```python
from build123d import *

# Parameters (mm, degrees)
SKETCH1_W           = 18
SKETCH1_H           = 28
SKETCH1_W_2         = 13
SKETCH1_H_2         = 16.2
BOSS_EXTRUDE1_DEPTH = 3
SKETCH1_3_W         = 13
SKETCH1_3_H         = 16.2
CUT_EXTRUDE1_DEPTH  = 17.911534525
SKETCH2_W           = 16.25
SKETCH2_H           = 19.6
CUT_EXTRUDE2_DEPTH  = 2
SKETCH4_W           = 10
SKETCH4_H           = 9
CUT_EXTRUDE3_DEPTH  = 17.911534525


with BuildPart() as part:
    # Sketch1 → Boss-Extrude1 (new body)
    # profile 1 of 2: a face of its own
    with BuildSketch(Plane(origin=(0, 0, 0), x_dir=(1, 0, 0), z_dir=(0, 1, 0))):
        Rectangle(SKETCH1_W, SKETCH1_H)
        Rectangle(SKETCH1_W_2, SKETCH1_H_2, mode=Mode.SUBTRACT)
    # profile 2 of 2: a face of its own
    with BuildSketch(Plane(origin=(0, 0, 0), x_dir=(1, 0, 0), z_dir=(0, 1, 0))):
        Rectangle(SKETCH1_W_2, SKETCH1_H_2)
    extrude(amount=BOSS_EXTRUDE1_DEPTH)

    # Sketch1<3> → Cut-Extrude1 (cut, through all)
    with BuildSketch(Plane(origin=(0, 0, 0), x_dir=(1, 0, 0), z_dir=(0, 1, 0))):
        Rectangle(SKETCH1_3_W, SKETCH1_3_H)
    extrude(amount=CUT_EXTRUDE1_DEPTH, mode=Mode.SUBTRACT)

    # Sketch2 → Cut-Extrude2 (cut)
    with BuildSketch(Plane(origin=(0, 3, 0), x_dir=(1, 0, 0), z_dir=(0, 1, 0))):
        Rectangle(SKETCH2_W, SKETCH2_H)
    extrude(amount=-CUT_EXTRUDE2_DEPTH, mode=Mode.SUBTRACT)

    # Sketch4 → Cut-Extrude3 (cut, through all)
    with BuildSketch(Plane(origin=(0, 3, 0), x_dir=(1, 0, 0), z_dir=(0, 1, 0))):
        with Locations((0, 9.8)):
            Rectangle(SKETCH4_W, SKETCH4_H)
    extrude(amount=-CUT_EXTRUDE3_DEPTH, mode=Mode.SUBTRACT)


solid = part.part
```
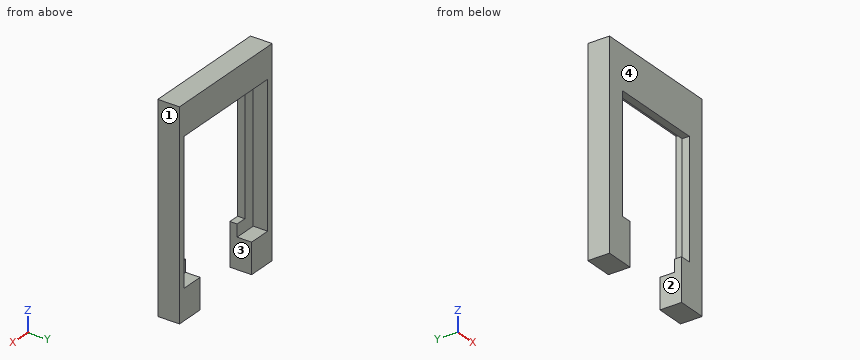
Verification items for the finished model (mm, model axes). Face numbers are marked on the shaded views. Give positions to 0.01 mm unless a question says otherwise; leave off trailing zeros. Order: outer loops, then holes, each group sorted by start corner. A loop starts at its lowest first (then second) coordinate and runs counter-clockwise, first axis right, second up. Notation, with made-up numbers: (81, 31) -> (122, 31) arc R22 cw to (122, 44) -> close; hole circle Ø10 at (-20, 79.5). An arc over 180 degrees is marked (long way). Use a Markdown table: item, result.
1) Section check C-C, the plane y = 2.2. Record the boundary of the cut face in (x, z) (3 decimals).
Results:
| item | result |
|---|---|
| outline | (-9, -14) -> (-5, -14) -> (-5, -9.8) -> (-8.125, -9.8) -> (-8.125, 9.8) -> (8.125, 9.8) -> (8.125, -9.8) -> (5, -9.8) -> (5, -14) -> (9, -14) -> (9, 14) -> (-9, 14) -> close |
2) Depth check by flat-ended pin: pin 1 Ø1.1 at (x, y) = (0, 0.5) entering from -Z; pin 2 Ø1.5 at (x, z) = (-5.5, -8.5) entering from +Y; pin 3 Ø1.6 at (x, y) = (2.5, 2) entering from -Z; pin 4 Ø1 at (x, z) = (4, -7.5) entering from -Y. Enter the tip coordinate at first touch or a pass-through.
Results:
| item | result |
|---|---|
| pin 1 | z = 8.1 |
| pin 2 | y = 1 |
| pin 3 | z = 9.8 |
| pin 4 | through |
3) Section check B-B, the plane x = -5.75. Record the boundary of the cut face in (y, z), then the cut area to 3 significant figures.
Results:
| item | result |
|---|---|
| outline | (0, -14) -> (3, -14) -> (3, -9.8) -> (1, -9.8) -> (1, -8.1) -> (0, -8.1) -> close; (0, 8.1) -> (1, 8.1) -> (1, 9.8) -> (3, 9.8) -> (3, 14) -> (0, 14) -> close |
| area | 28.6 mm² |
4) Mould release check, pull along X, two halves, no side actions. Record for the marked faces 1, 2, 3 and 4: pulls with the +X half, pulls with the -X half, needs draft (parallel to the pull), parting line crosses it, or undercut.
Results:
| item | result |
|---|---|
| face 1 | pulls with the +X half |
| face 2 | undercut |
| face 3 | undercut |
| face 4 | needs draft |
5) Section check D-D, the plane x = 2.5. Record the boundary of the cut face in (y, z), then the cut area to 3 significant figures.
Results:
| item | result |
|---|---|
| outline | (0, 8.1) -> (1, 8.1) -> (1, 9.8) -> (3, 9.8) -> (3, 14) -> (0, 14) -> close |
| area | 14.3 mm² |
6) Material ranges on probe 1 along Z at (x, y) = (7.5, 1.3); probe 2 along X at (y, z) = (0.6, 0.5); probe 3 along Z at (x, y) = (-6, 0.6), recorded low to high.
Results:
| item | result |
|---|---|
| probe 1 | -14 to -9.8, 9.8 to 14 |
| probe 2 | -9 to -6.5, 6.5 to 9 |
| probe 3 | -14 to -8.1, 8.1 to 14 |
7) Section check A-A, the plane z = -4.5. Record the boundary of the cut face in (x, y) (3 decimals), then the cut area to 3 significant figures.
Results:
| item | result |
|---|---|
| outline | (-9, 0) -> (-6.5, 0) -> (-6.5, 1) -> (-8.125, 1) -> (-8.125, 3) -> (-9, 3) -> close; (6.5, 0) -> (9, 0) -> (9, 3) -> (8.125, 3) -> (8.125, 1) -> (6.5, 1) -> close |
| area | 8.50 mm² |
